The model under review builds one solid part; all positions refer to its coordinate system, in mm. A direction names the side the tool comes from. Coordinates: 2 decimals unless noted, no trailing zeros. Write each loop counter-clockwise with the first axis right and the second up, starting at its lowest first coordinate (ties: lowest second). Pieces come first, ordered by that corner, then holes. Notation, with made-up numbers: M 39,37 L 83,37 A20 ccw 83,72 Z; hole C -19.75,79.25 d9. An arc over 180 degrees is marked long. Answer as a JSON object with one key per item and string values.
```python
from build123d import *

# Parameters (mm, degrees)
SKETCH1_R               = 5
SKETCH1_R_2             = 4
BOSS_EXTRUDE1_DEPTH     = 50
CUT_EXTRUDE1_DEPTH      = 52
CUT_EXTRUDE1_DEPTH_BACK = 35
SKETCH2_W               = 30
SKETCH2_H               = 80
SKETCH3_W               = 30
SKETCH3_H               = 40
CUT_EXTRUDE2_DEPTH      = 52
CUT_EXTRUDE3_START      = -10
CUT_EXTRUDE3_DEPTH      = 30
CUT_EXTRUDE4_START      = -10
CUT_EXTRUDE4_DEPTH      = 30
FILLET1_R               = 10
SKETCH7_R               = 6.5
CUT_EXTRUDE5_DEPTH      = 5
CUT_EXTRUDE6_START      = -5
SKETCH6_R               = 6.5
CUT_EXTRUDE6_DEPTH      = 5
SKETCH8_R               = 3
CUT_EXTRUDE8_DEPTH      = 16


with BuildPart() as part:
    # Sketch1 → Boss-Extrude1 (new body)
    with BuildSketch(Plane(origin=(0, 0, 0), x_dir=(0, 0, -1), z_dir=(1, 0, 0))):
        with BuildLine():
            Line((-255.87149894, 42.046001407), (44.12850106, 42.046001407))
            add(Edge.make_bspline(
                [(44.12850106, 42.046001407), (144.12850106, 17.046001407), (44.12850106, -7.953998593)],
                knots=[0, 0, 0, 1, 1, 1], degree=2))
            Line((44.12850106, -7.953998593), (-255.87149894, -7.953998593))
            add(Edge.make_bspline(
                [(-255.87149894, 42.046001407), (-335.87149894, 17.046001407), (-255.87149894, -7.953998593)],
                knots=[0, 0, 0, 1, 1, 1], degree=2))
        make_face()
        with Locations((-280.87149894, 17.046001407)):
            Circle(SKETCH1_R, mode=Mode.SUBTRACT)
        with Locations((69.12850106, 17.046001407)):
            Circle(SKETCH1_R_2, mode=Mode.SUBTRACT)
    extrude(amount=BOSS_EXTRUDE1_DEPTH)

    # Sketch2 → Cut-Extrude1 (cut, two sides: drawn at the far end of the back side and taken through both)
    with BuildSketch(Plane(origin=(0, 0, 0), x_dir=(1, 0, 0), z_dir=(0, 1, 0)).offset(-CUT_EXTRUDE1_DEPTH_BACK)):
        with Locations((25, 54.12850106)):
            Rectangle(SKETCH2_W, SKETCH2_H)
    extrude(amount=CUT_EXTRUDE1_DEPTH + CUT_EXTRUDE1_DEPTH_BACK, mode=Mode.SUBTRACT)

    # Sketch3 → Cut-Extrude2 (cut)
    with BuildSketch(Plane.XZ.offset(7.953998593)):
        with Locations((25, 275.87149894)):
            Rectangle(SKETCH3_W, SKETCH3_H)
    extrude(amount=-CUT_EXTRUDE2_DEPTH, mode=Mode.SUBTRACT)

    # Sketch4 → Cut-Extrude3 (cut)
    with BuildSketch(Plane.ZY.offset(CUT_EXTRUDE3_START)):
        Polygon((-14.12850106, 17.046001407), (-14.12850106, 42.046001407), (29.172769129, 42.046001407), align=None)
    extrude(amount=-CUT_EXTRUDE3_DEPTH, mode=Mode.SUBTRACT)

    # Sketch5 → Cut-Extrude4 (cut)
    with BuildSketch(Plane.ZY.offset(CUT_EXTRUDE4_START)):
        Polygon((-14.12850106, -7.953998593), (-14.12850106, 17.046001407), (29.172769129, -7.953998593), align=None)
    extrude(amount=-CUT_EXTRUDE4_DEPTH, mode=Mode.SUBTRACT)

    # Fillet1
    fillet1_edges = [part.edges().sort_by_distance(p)[0] for p in [
        (25, 17.046001407, -14.12850106),
    ]]
    fillet(fillet1_edges, radius=FILLET1_R)

    # Sketch7 → Cut-Extrude5 (cut)
    with BuildSketch(Plane.ZY.offset(-40)):
        with Locations((-69.12850106, 17.046001407)):
            Circle(SKETCH7_R)
    extrude(amount=-CUT_EXTRUDE5_DEPTH, mode=Mode.SUBTRACT)

    # Sketch6 → Cut-Extrude6 (cut)
    with BuildSketch(Plane(origin=(10, 0, 0), x_dir=(0, 0, -1), z_dir=(1, 0, 0)).offset(CUT_EXTRUDE6_START)):
        with Locations(Location((69.12850106, 17.046001407, 0), (0, 0, 180))):
            Circle(SKETCH6_R)
    extrude(amount=CUT_EXTRUDE6_DEPTH, mode=Mode.SUBTRACT)

    # Sketch8 → Cut-Extrude8 (cut)
    with BuildSketch(Plane.ZY):
        with Locations(Location((15.87149894, 7.046001407, 0), (0, 0, 180))):
            Circle(SKETCH8_R)
        with Locations((15.87149894, 27.046001407)):
            Circle(SKETCH8_R)
    extrude(amount=-CUT_EXTRUDE8_DEPTH, mode=Mode.SUBTRACT)


solid = part.part
```
(1) Add section B-B on x = 26.5. Give the boundary of the cut face in (y, z), and give its area (3 significant figures).
Results list:
{"outline": "M -7.95,29.17 L 8.39,0.87 A10 ccw 25.71,0.87 L 42.05,29.17 L 42.05,255.87 L -7.95,255.87 Z", "area": "12,300 mm²"}
(2) Wall thickness on line 1 along X through (y, z) = (25, -75.5); line 2 along Z through (x, y) = (46.5, 15); line 3 along Y through (x, z) = (44, -59.5): over which ranges is each line inside the solid? List them lowest first. Write a range as from..to.
Results list:
{"line 1": "0..10, 40..50", "line 2": "-93.79..-72.57, -65.69..276.31, 285.43..295.6", "line 3": "-3.76..37.85"}
(3) Add section A-A on z = -31. Give the boundary of the cut face in (x, y).
Results list:
{"outline": "M 0,-7.95 L 10,-7.95 L 10,42.05 L 0,42.05 Z; M 40,-7.95 L 50,-7.95 L 50,42.05 L 40,42.05 Z"}
(4) For pin 1 Ø12 at (x, y) = (32, 22) entering from -Z; pin 2 Ø4 at (x, y) = (28, 34) entering from +Z; pin 3 Ø5 at (y, z) = (17.05, -69.13) entering from +X, all flat-tipped, find the tip position at first contact; note any pin that passes through.
Results list:
{"pin 1": "z = -4.13", "pin 2": "z = 255.87", "pin 3": "through"}
(5) Draft analysis for pull direction Z (two halves, no side actions). For faces 5 (the face through (5, 14, -66)), 6 (the face through (25, 17, 255.871)), 7 (the face through (40, 17, 271)), state which applies: released by +Z, released by -Z, zero draft, split by the parting line, or undercut.
Results list:
{"face 5": "undercut", "face 6": "released by +Z", "face 7": "zero draft"}
(6) For faces 1 (the face through (7.465, 19.536, -63.124)), 2 (the face through (25.21, 16.899, -4.127)), 3 (the face through (24.79, 33.99, 15.22)), 4 (the face through (10, 17, 271)), list the 3-axis set-ups (+Z, -Z, +X, -X, +Y, -Y) from which the entire face can be reached by the end or side of a thin tool; tool diameter is ignored.
Results list:
{"face 1": "none", "face 2": "-Z", "face 3": "-Z, +Y", "face 4": "+Z, +Y, -Y"}
